```python
from build123d import *

# Parameters (mm, degrees)
F0_R     = 23.5
F1_DEPTH = 80.8
F2_R     = 21.5
F3_DEPTH = 3.4
F5_R     = 15.425
F6_DEPTH = 3.5
F7_R     = 14.25
F8_DEPTH = 77.301
F4_R     = 21
F9_DEPTH = 71.9


with BuildPart() as f1:
    # F0 (on Top) → F1 (new body)
    with BuildSketch(Plane.XY):
        Circle(F0_R)
    extrude(amount=F1_DEPTH)

    # F2 (on face) → F3 (cut)
    with BuildSketch(Plane.XY.offset(80.8)):
        Circle(F2_R)
    extrude(amount=-F3_DEPTH, mode=Mode.SUBTRACT)

    # F5 (on face) → F6 (cut)
    with BuildSketch(Plane(origin=(0, 0, 0), x_dir=(1, 0, 0), z_dir=(0, 0, -1))):
        Circle(F5_R)
    extrude(amount=-F6_DEPTH, mode=Mode.SUBTRACT)

    # F7 (on face) → F8 (cut, through all)
    with BuildSketch(Plane(origin=(0, 0, 3.5), x_dir=(1, 0, 0), z_dir=(0, 0, -1))):
        Circle(F7_R)
    extrude(amount=-F8_DEPTH, mode=Mode.SUBTRACT)

    # F4 (on face) → F9 (cut, through all)
    with BuildSketch(Plane.XY.offset(77.4)):
        Circle(F4_R)
    extrude(amount=-F9_DEPTH, mode=Mode.SUBTRACT)


solid = f1.part
```
Source: CAD feature listing. Evaluate the final solid. Frame: model axes, mm. A direction names the side the tool comes from. Give positions to 0.01 mm unless a question says otherwise; leave off trailing zeros. Order: outer loops, then holes, each group sorted by start corner. A loop starts at its lowest first (then second) coordinate and runs counter-clockwise, first axis right, second up.
(1) Pull-direction query (Y, two-part tool) for faces 4 (the face through (5, -15, 0)), 5 (the face through (22.4, 7.1, 39.8)), 6 (the face through (13.163, 5.458, 4.486)); classes: +Y half, -Y half, draft (parallel to the pull), parting line (faces both ways), or undercut.
(2) Section query A-A (y = 0). Return the cut outline in (x, z) (3 decimals), plus the area to 3 significant figures.
(3) Material intervals for line 1 along Y through (x, z) = (0, 27.5); line 2 along Y through (x, z) = (0, 1.6) (3 decimals); line 3 along X through (y, z) = (10.5, 46.5), sorted ascending.
(4) Section query C-C (z = 28). Return the cut outline in (x, y).
(5) Access query for faces 1 (the face through (4, 14, 3.5)), 2 (the face through (19, -9.5, 77.4)), 3 (the face through (10.33, -19.04, 80.8)). Directions: +Z, -Z, +X, -X, +Y, -Y. A direction counts if a zero-diameter tool reaches every point of the face in a straight line with its end or side. Return the directions, or none.
(6) Contact query for flat-ended pins moving along their axis: P1, Ø10, axis at x = -4.5, z = 71.5, coming from the +Y side; P2, Ø4, axis at x = 13.5, z = 10, coming from the -Y side; P3, Ø24.5, axis at x = 1.5, y = -3, coming from the -Z side; P4, Ø3, axis at x = 10.5, z = 37.5, coming from the -Y side. Output: stop coordinate, or through.
Outcome:
1. face 4: draft
1. face 5: parting line
1. face 6: undercut
2. outline: (-23.5, 0) - (-15.425, 0) - (-15.425, 3.5) - (-14.25, 3.5) - (-14.25, 5.5) - (-21, 5.5) - (-21, 77.4) - (-21.5, 77.4) - (-21.5, 80.8) - (-23.5, 80.8) - close; (14.25, 3.5) - (15.425, 3.5) - (15.425, 0) - (23.5, 0) - (23.5, 80.8) - (21.5, 80.8) - (21.5, 77.4) - (21, 77.4) - (21, 5.5) - (14.25, 5.5) - close
2. area: 467 mm2
3. line 1: y = -23.5 to -21, 21 to 23.5
3. line 2: y = -23.5 to -15.425, 15.425 to 23.5
3. line 3: x = -21.02 to -18.19, 18.19 to 21.02
4. outline: circle Ø47 at (0, 0); hole circle Ø42 at (0, 0)
5. face 1: -Z
5. face 2: +Z
5. face 3: +Z, +X, -X, +Y, -Y
6. P1: stops at y = 23.5
6. P2: stops at y = -20.49
6. P3: stops at z = 0
6. P4: stops at y = -21.71
